```python
from build123d import *

# Parameters (mm, degrees)
SKETCH1_W           = 87
SKETCH1_H           = 7
BOSS_EXTRUDE1_DEPTH = 66
FILLET1_R           = 6
SKETCH2_R           = 5
CUT_EXTRUDE1_DEPTH  = 111.675200474
SKETCH3_R           = 9.5
BOSS_EXTRUDE2_DEPTH = 13
SKETCH9_R           = 14


with BuildPart() as part:
    # Sketch1 → Boss-Extrude1 (new body)
    with BuildSketch(Plane.XY):
        with Locations((43.5, 3.5)):
            Rectangle(SKETCH1_W, SKETCH1_H)
        with BuildLine():
            ThreePointArc((35, 0), (38.535533906, -1.464466094), (40, -5))
            Line((40, -5), (40, -11))
            Line((40, -11), (87, -11))
            Line((87, -11), (87, 0))
            Line((87, 0), (35, 0))
        make_face()
    extrude(amount=BOSS_EXTRUDE1_DEPTH)

    # Fillet1
    fillet1_edges = [part.edges().sort_by_distance(p)[0] for p in [
        (43.5, 7, 66),
        (43.5, 7, 0),
    ]]
    fillet(fillet1_edges, radius=FILLET1_R)

    # Sketch2 → Cut-Extrude1 (cut, through all)
    with BuildSketch(Plane(origin=(0, 7, 0), x_dir=(1, 0, 0), z_dir=(0, 1, 0))):
        with Locations(Location((50.635865221, -47, 0), (0, 0, 270))):
            Circle(SKETCH2_R)
        with Locations(Location((17.635865221, -47, 0), (0, 0, 270))):
            Circle(SKETCH2_R)
        with Locations(Location((50.635865221, -19, 0), (0, 0, 90))):
            Circle(SKETCH2_R)
        with Locations(Location((17.635865221, -19, 0), (0, 0, 270))):
            Circle(SKETCH2_R)
    extrude(amount=-CUT_EXTRUDE1_DEPTH, mode=Mode.SUBTRACT)

    # Sketch3 → Boss-Extrude2 (add)
    with BuildSketch(Plane(origin=(87, 0, 0), x_dir=(0, 0, -1), z_dir=(1, 0, 0))):
        with BuildLine():
            Line((0, -11), (-66, -11))
            Line((-66, -11), (-53.656311688, -36.45938769))
            ThreePointArc((-53.656311688, -36.45938769), (-33.320230855, -49.283211846), (-12.834921269, -36.699144903))
            Line((-12.834921269, -36.699144903), (0, -11))
        make_face()
        with Locations((-33, -27)):
            Circle(SKETCH3_R, mode=Mode.SUBTRACT)
    extrude(amount=-BOSS_EXTRUDE2_DEPTH)

    # Cut-Sweep4: sweep along a path in Sketch8
    with BuildLine(Plane.XY.offset(33)) as cut_sweep4_path:
        Line((87, -7), (62, 7))
    # Sketch9 → Cut-Sweep4 (sweep, cut)
    with BuildSketch(Plane(origin=(87, 0, 0), x_dir=(0, 0, -1), z_dir=(1, 0, 0))):
        with Locations((-33, 7)):
            Circle(SKETCH9_R)
    sweep(path=cut_sweep4_path.line, mode=Mode.SUBTRACT)


solid = part.part
```
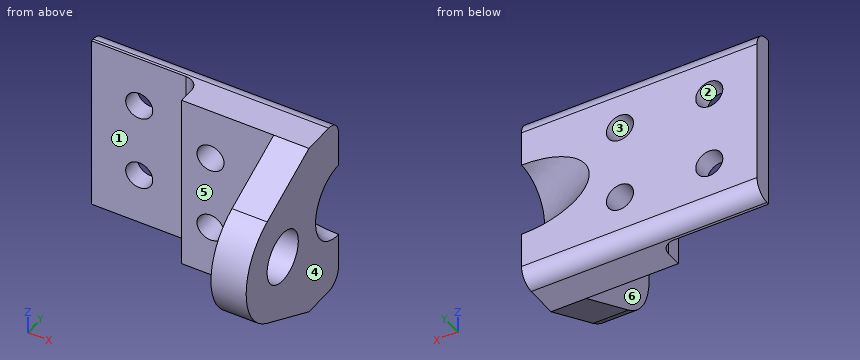
The listing builds one solid part. Answer for the finished solid, in the listing's coordinates (mm). Face numbers are marked on the shaded views. A direction names the side the tool comes from. Round coordinates to 2 decimals unless told otherwise and drop trailing zeros. Write each loop counter-clockwise with the first axis right and the second up, starting at its lowest first coordinate (ties: lowest second). Pieces come first, ordered by that corner, then holes. Notation, with made-up numbers: (24.25, 8.25) -> (68.25, 8.25) arc R18 ccw to (68.25, 18.25) -> close; hole circle Ø4 at (-5.5, 82). An arc over 180 degrees is marked (long way). Write item = value, one per line.
1) Section C-C on x = 30 is taken. Write down the section's boundary in (y, z), plus the area to 3 significant figures.
Check values:
outline = (0, 0) -> (1, 0) arc R6 ccw to (7, 6) -> (7, 60) arc R6 ccw to (1, 66) -> (0, 66) -> close
area = 447 mm²
2) Section D-D on y = -34.5 is taken. Write down the section's boundary in (x, z), plus the area to 3 significant figures.
Check values:
outline = (74, 11.74) -> (87, 11.74) -> (87, 27.17) -> (74, 27.17) -> close; (74, 38.83) -> (87, 38.83) -> (87, 54.61) -> (74, 54.61) -> close
area = 406 mm²
3) Straight lines are drawn through the part: line 1 along X through (y, z) = (1.75, 47); line 2 along Z through (x, y) = (18.5, 3.5); line 3 along X through (y, z) = (-31, 54). For each, find the intervals that lie inside material, in ascending order. Write a range as [from, to].
Check values:
line_1 = [0, 12.64], [22.64, 45.64], [55.64, 87]
line_2 = [0.55, 14.08], [23.92, 42.08], [51.92, 65.45]
line_3 = [74, 87]
4) Given pin 1 (11.5 mm diameter, centred on y = -32, z = 29, fed in from -X); pin 2 (1.8 mm diameter, centred on y = -7.5, z = 21, fed in from -X); pin 3 (10 mm diameter, centred on x = 62.5, z = 48.5, fed in from -Y), each flat-ended and moving along its own axis, determine where each tip first touches the part or whether it passes through.
Check values:
pin_1 = 74
pin_2 = 40
pin_3 = -11
5) Section B-B on y = -27 is taken. Write down the section's boundary in (x, z).
Check values:
outline = (74, 7.99) -> (87, 7.99) -> (87, 23.5) -> (74, 23.5) -> close; (74, 42.5) -> (87, 42.5) -> (87, 58.24) -> (74, 58.24) -> close
6) Which of the six approach directions +Z, -Z, +X, -X, +Y, -Y give full straight-line access (tool end or side, diameter ignored) to the marked faces 1 and 2?
Check values:
face_1 = +Z, -Z, -X, -Y
face_2 = +Y, -Y
7) For a pull along X with two mould halves and no side action, classify the marked faces 3, 4, 5 and 6 as released by +X, released by -X, zero draft, split by the parting line, or undercut.
Check values:
face_3 = undercut
face_4 = released by +X
face_5 = zero draft
face_6 = released by -X
8) Section A-A on x = 52 is taken. Write down the section's boundary in (y, z), plus the area to 3 significant figures.
Check values:
outline = (-11, 0) -> (1, 0) arc R6 ccw to (7, 6) -> (7, 14.19) -> (-11, 14.19) -> close; (-11, 23.81) -> (7, 23.81) -> (7, 42.19) -> (-11, 42.19) -> close; (-11, 51.81) -> (7, 51.81) -> (7, 60) arc R6 ccw to (1, 66) -> (-11, 66) -> close
area = 826 mm²
